Input: dimensioned drawing with shaded views. Units: mm. Origin: part minimum x, y, z. Give positions to 0.01 mm unless a question says otherwise; leave off trailing zeros. Loops run counter-clockwise (first coordinate to the right, second up) from the corner with the lowest first, then second, coordinate; pieces in that order, holes last. Notation, with made-up numbers: (57.25, -6) -> (111.25, -6) arc R10 cw to (111.25, 3) -> close; hole circle Ø8 at (-14, 84.5). An arc over 180 degrees is marked (long way). Answer in a Markdown table with one row per item. Add a question column.
1) Section query B-B (x = 10.75). Return the cut outline in (y, z).
2) Line query: line 1 (Y direction, x = 10.75, z = 0.4); line 2 (X direction, y = 9, z = 0.65) (1 decimal); line 3 (Z direction, x = 26, y = 14.5). Output: solid intervals per line, ascending. Write a range as from..to.
3) Section query C-C (y = 3.25). Return the cut outline in (x, z).
4) Section query A-A (z = 2.4). Return the cut outline in (x, y), plus the area to 3 significant figures.
5) First-contact query: P1, Ø3.5, axis at x = 11.5, y = 12.5, coming from the +Z side; P2, Ø1, axis at x = 23, y = 10, coming from the +Z side. Flat tips, straight axial feed; report the tip coordinate or a pass-through.
6) Section query D-D (y = 9.5). Give the number of separate pieces and of enclosed holes in the cut face.
7) Draft query along X for the marked faces 1, 2 and 3. Return one class per face: +X half, -X half, draft (parallel to the pull), parting line (faces both ways), or undercut.
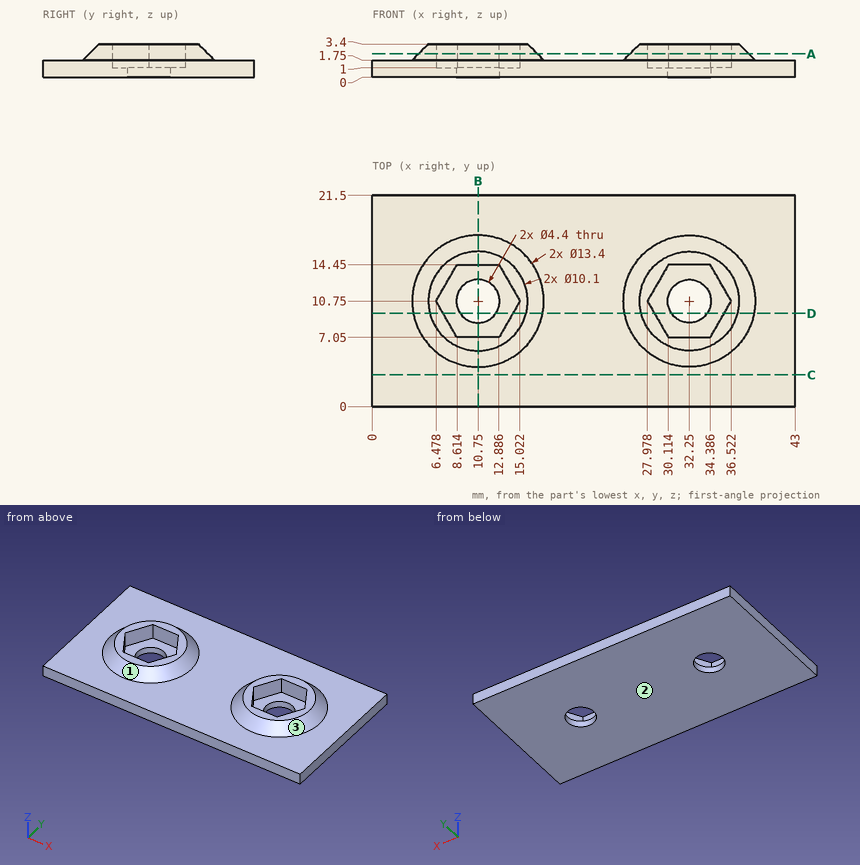
Evaluation:
| question | item | result |
|---|---|---|
| 1 | outline | (0, 0) -> (8.55, 0) -> (8.55, 1) -> (7.05, 1) -> (7.05, 3.4) -> (5.7, 3.4) -> (4.05, 1.75) -> (0, 1.75) -> close; (12.95, 0) -> (21.5, 0) -> (21.5, 1.75) -> (17.45, 1.75) -> (15.8, 3.4) -> (14.45, 3.4) -> (14.45, 1) -> (12.95, 1) -> close |
| 2 | line 1 | 0..8.55, 12.95..21.5 |
| 2 | line 2 | 0..9.4, 12.1..30.9, 33.6..43 |
| 2 | line 3 | 0..1.75 |
| 3 | outline | (0, 0) -> (43, 0) -> (43, 1.75) -> (0, 1.75) -> close |
| 4 | outline | circle Ø12.1 at (10.75, 10.75); circle Ø12.1 at (32.25, 10.75); hole (6.48, 10.75) -> (8.61, 7.05) -> (12.89, 7.05) -> (15.02, 10.75) -> (12.89, 14.45) -> (8.61, 14.45) -> close; hole (27.98, 10.75) -> (30.11, 7.05) -> (34.39, 7.05) -> (36.52, 10.75) -> (34.39, 14.45) -> (30.11, 14.45) -> close |
| 4 | area | 135 mm² |
| 5 | P1 | z = 1 |
| 5 | P2 | z = 1.75 |
| 6 | separate pieces | 3 |
| 6 | enclosed holes | 0 |
| 7 | face 1 | undercut |
| 7 | face 2 | draft |
| 7 | face 3 | undercut |
